from build123d import *

# Parameters (mm, degrees)
SKETCH_1_R          = 1.6
SKETCH_1_R_2        = 1.65
EXTRUDE_1_DEPTH     = 5
FILLET_1_R          = 2
SKETCH_2_R          = 3.5
CUT_EXTRUDE_1_DEPTH = 2.5
SKETCH_3_W          = 15.1
SKETCH_3_H          = 85
CUT_EXTRUDE_2_DEPTH = 1
SKETCH_4_R          = 1.25
CUT_EXTRUDE_3_DEPTH = 5
CHAMFER_1_SIZE      = 5
SKETCH_6_R          = 1.25
CUT_EXTRUDE_5_DEPTH = 5
SKETCH_7_R          = 1.25
CUT_EXTRUDE_6_DEPTH = 5
SKETCH_5_R          = 2.1
CUT_EXTRUDE_4_DEPTH = 6
CUT_EXTRUDE_7_DEPTH = 2.5
CUT_EXTRUDE_9_DEPTH = 6.0000001
SKETCH_9_W          = 33.95
SKETCH_9_H          = 29
CUT_EXTRUDE_8_DEPTH = 3.5
FILLET_29_R         = 2.1
FILLET_30_R         = 2


with BuildPart() as part:
    # ｽｹｯﾁ1 → ﾎﾞｽ - 押し出し1 (new body)
    with BuildSketch(Plane(origin=(0, 0, 0), x_dir=(1, 0, 0), z_dir=(0, 1, 0))):
        Polygon((-36.5, -42.5), (31.5, -42.5), (36.5, -32.5), (36.5, 32.5), (31.5, 42.5), (-36.5, 42.5), align=None)
        with Locations((-24, -18)):
            Circle(SKETCH_1_R, mode=Mode.SUBTRACT)
        with Locations((-24, 18)):
            Circle(SKETCH_1_R, mode=Mode.SUBTRACT)
        with Locations((24, 35)):
            Circle(SKETCH_1_R_2, mode=Mode.SUBTRACT)
        with Locations((24, -35)):
            Circle(SKETCH_1_R_2, mode=Mode.SUBTRACT)
        with Locations((24, -18)):
            Circle(SKETCH_1_R, mode=Mode.SUBTRACT)
        with Locations((24, 18)):
            Circle(SKETCH_1_R, mode=Mode.SUBTRACT)
    extrude(amount=EXTRUDE_1_DEPTH)

    # ﾌｨﾚｯﾄ1
    fillet_1_edges = [part.edges().sort_by_distance(p)[0] for p in [
        (31.5, 2.5, -42.5),
        (36.5, 2.5, -32.5),
        (36.5, 2.5, 32.5),
        (31.5, 2.5, 42.5),
    ]]
    fillet(fillet_1_edges, radius=FILLET_1_R)

    # ｽｹｯﾁ2 → ｶｯﾄ - 押し出し1 (cut)
    with BuildSketch(Plane(origin=(0, 5, 0), x_dir=(1, 0, 0), z_dir=(0, 1, 0))):
        with Locations((24, 18)):
            Circle(SKETCH_2_R)
        with Locations((24, -18)):
            Circle(SKETCH_2_R)
    extrude(amount=-CUT_EXTRUDE_1_DEPTH, mode=Mode.SUBTRACT)

    # ｽｹｯﾁ3 → ｶｯﾄ - 押し出し2 (cut)
    with BuildSketch(Plane(origin=(0, 5, 0), x_dir=(1, 0, 0), z_dir=(0, 1, 0))):
        with Locations((24, 0)):
            Rectangle(SKETCH_3_W, SKETCH_3_H)
    extrude(amount=-CUT_EXTRUDE_2_DEPTH, mode=Mode.SUBTRACT)

    # ｽｹｯﾁ4 → ｶｯﾄ - 押し出し3 (cut)
    with BuildSketch(Plane.ZY.offset(36.5)):
        with Locations((-35, 2.5)):
            Circle(SKETCH_4_R)
        with Locations((35, 2.5)):
            Circle(SKETCH_4_R)
    extrude(amount=-CUT_EXTRUDE_3_DEPTH, mode=Mode.SUBTRACT)

    # 面取り1
    chamfer_1_edges = [part.edges().sort_by_distance(p)[0] for p in [
        (-36.5, 2.5, 42.5),
        (-36.5, 2.5, -42.5),
    ]]
    chamfer(chamfer_1_edges, length=CHAMFER_1_SIZE)

    # ｽｹｯﾁ6 → ｶｯﾄ - 押し出し5 (cut)
    with BuildSketch(Plane.XY.offset(42.5)):
        with Locations((8.5, 2.5)):
            Circle(SKETCH_6_R)
    extrude(amount=-CUT_EXTRUDE_5_DEPTH, mode=Mode.SUBTRACT)

    # ｽｹｯﾁ7 → ｶｯﾄ - 押し出し6 (cut)
    with BuildSketch(Plane(origin=(0, 0, -42.5), x_dir=(-1, 0, 0), z_dir=(0, 0, -1))):
        with Locations((-8.5, 2.5)):
            Circle(SKETCH_7_R)
    extrude(amount=-CUT_EXTRUDE_6_DEPTH, mode=Mode.SUBTRACT)

    # ｽｹｯﾁ5 → ｶｯﾄ - 押し出し4 (cut, through all)
    with BuildSketch(Plane(origin=(0, 5, 0), x_dir=(1, 0, 0), z_dir=(0, 1, 0))):
        with Locations((-38.5, 35)):
            Circle(SKETCH_5_R)
        with Locations((-38.5, -35)):
            Circle(SKETCH_5_R)
        with Locations((8.5, -44.5)):
            Circle(SKETCH_5_R)
        with Locations((8.5, 44.5)):
            Circle(SKETCH_5_R)
    extrude(amount=-CUT_EXTRUDE_4_DEPTH, mode=Mode.SUBTRACT)

    # ｽｹｯﾁ8 → ｶｯﾄ - 押し出し7 (cut)
    with BuildSketch(Plane(origin=(0, 5, 0), x_dir=(1, 0, 0), z_dir=(0, 1, 0))):
        with BuildLine():
            Line((-20.5, 18), (-20.5, 21.5))
            Line((-20.5, 21.5), (-24, 21.5))
            ThreePointArc((-24, 21.5), (-26.474873734, 20.474873734), (-27.5, 18))
            Line((-27.5, 18), (-27.5, 14.5))
            Line((-27.5, 14.5), (-24, 14.5))
            ThreePointArc((-24, 14.5), (-21.525126266, 15.525126266), (-20.5, 18))
        make_face()
        with BuildLine():
            Line((-27.5, -18), (-27.5, -14.5))
            Line((-27.5, -14.5), (-24, -14.5))
            ThreePointArc((-24, -14.5), (-21.525126266, -15.525126266), (-20.5, -18))
            Line((-20.5, -18), (-20.5, -21.5))
            Line((-20.5, -21.5), (-24, -21.5))
            ThreePointArc((-24, -21.5), (-26.474873734, -20.474873734), (-27.5, -18))
        make_face()
    extrude(amount=-CUT_EXTRUDE_7_DEPTH, mode=Mode.SUBTRACT)

    # ｽｹｯﾁ10 → ｶｯﾄ - 押し出し9 (cut, through all)
    with BuildSketch(Plane(origin=(0, 5, 0), x_dir=(1, 0, 0), z_dir=(0, 1, 0))):
        with BuildLine():
            Line((-31.5, 32.5), (-31.5, 37.5))
            ThreePointArc((-31.5, 37.5), (-30, 39), (-28.5, 37.5))
            Line((-28.5, 37.5), (-28.5, 32.5))
            ThreePointArc((-28.5, 32.5), (-30, 31), (-31.5, 32.5))
        make_face()
        with BuildLine():
            Line((6, 37.5), (11, 37.5))
            ThreePointArc((11, 37.5), (12.5, 36), (11, 34.5))
            Line((11, 34.5), (6, 34.5))
            ThreePointArc((6, 34.5), (4.5, 36), (6, 37.5))
        make_face()
        with BuildLine():
            Line((6, -37.5), (11, -37.5))
            ThreePointArc((11, -37.5), (12.5, -36), (11, -34.5))
            Line((11, -34.5), (6, -34.5))
            ThreePointArc((6, -34.5), (4.5, -36), (6, -37.5))
        make_face()
        with BuildLine():
            Line((-31.5, -32.5), (-31.5, -37.5))
            ThreePointArc((-31.5, -37.5), (-30, -39), (-28.5, -37.5))
            Line((-28.5, -37.5), (-28.5, -32.5))
            ThreePointArc((-28.5, -32.5), (-30, -31), (-31.5, -32.5))
        make_face()
    extrude(amount=-CUT_EXTRUDE_9_DEPTH, mode=Mode.SUBTRACT)

    # ｽｹｯﾁ9 → ｶｯﾄ - 押し出し8 (cut)
    with BuildSketch(Plane(origin=(0, 5, 0), x_dir=(1, 0, 0), z_dir=(0, 1, 0))):
        with Locations((-3.525, 0)):
            Rectangle(SKETCH_9_W, SKETCH_9_H)
        with BuildLine():
            Line((-24, 21.5), (13.45, 21.5))
            Line((13.45, 21.5), (13.45, 34.5))
            Line((13.45, 34.5), (13.45, 37.5))
            Line((13.45, 37.5), (11, 37.5))
            Line((11, 37.5), (6, 37.5))
            Line((6, 37.5), (4.5, 37.5))
            Line((4.5, 37.5), (2.5, 39.5))
            Line((2.5, 39.5), (-31.5, 39.5))
            Line((-31.5, 39.5), (-31.5, 37.5))
            Line((-31.5, 37.5), (-31.5, 32.5))
            Line((-31.5, 32.5), (-31.5, 31))
            Line((-31.5, 31), (-33.5, 29))
            Line((-33.5, 29), (-33.5, -29))
            Line((-33.5, -29), (-31.5, -31))
            Line((-31.5, -31), (-31.5, -32.5))
            Line((-31.5, -32.5), (-31.5, -37.5))
            Line((-31.5, -37.5), (-31.5, -39.5))
            Line((-31.5, -39.5), (2.5, -39.5))
            Line((2.5, -39.5), (4.5, -37.5))
            Line((4.5, -37.5), (6, -37.5))
            Line((6, -37.5), (11, -37.5))
            Line((11, -37.5), (13.45, -37.5))
            Line((13.45, -37.5), (13.45, -34.5))
            Line((13.45, -34.5), (13.45, -21.5))
            Line((13.45, -21.5), (-24, -21.5))
            ThreePointArc((-24, -21.5), (-26.474873734, -20.474873734), (-27.5, -18))
            Line((-27.5, -18), (-27.5, 18))
            ThreePointArc((-27.5, 18), (-26.474873734, 20.474873734), (-24, 21.5))
        make_face()
    extrude(amount=-CUT_EXTRUDE_8_DEPTH, mode=Mode.SUBTRACT)

    # ﾌｨﾚｯﾄ29
    fillet_29_edges = [part.edges().sort_by_distance(p)[0] for p in [
        (13.45, 3.25, -21.5),
        (4.5, 3.25, -37.5),
        (13.45, 3.25, 37.5),
        (-31.5, 3.25, -31),
        (13.45, 3.25, 21.5),
        (4.5, 3.25, 37.5),
        (2.5, 3.25, 39.5),
        (-31.5, 3.25, 31),
        (-33.5, 3.25, 29),
        (-33.5, 3.25, -29),
        (2.5, 3.25, -39.5),
        (13.45, 3.25, -37.5),
        (-20.5, 3.25, 14.5),
        (-20.5, 3.25, -14.5),
        (13.45, 3.25, -14.5),
        (13.45, 3.25, 14.5),
    ]]
    fillet(fillet_29_edges, radius=FILLET_29_R)

    # ﾌｨﾚｯﾄ30
    fillet_30_edges = [part.edges().sort_by_distance(p)[0] for p in [
        (-31.5, 3.25, 39.5),
        (-31.5, 3.25, -39.5),
    ]]
    fillet(fillet_30_edges, radius=FILLET_30_R)


solid = part.part
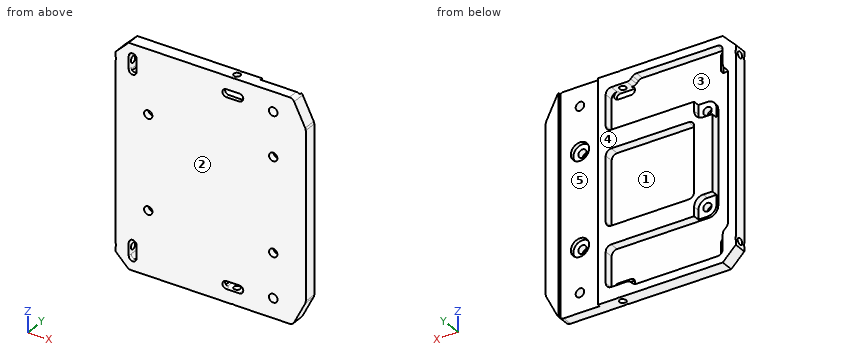
Geometry: final body of the model. Coordinates: model frame, mm. Face numbers are marked on the shaded views. A direction names the side the tool comes from. Round coordinates to 2 decimals unless told otherwise and drop trailing zeros. Loops run counter-clockwise (first coordinate to the right, second up) from the corner with the lowest first, then second, coordinate; pieces in that order, holes last.
Q1. Section A-A on z = 7.5. Return loops of the section in (x, y).
Q2. Pull-direction query (X, two-part tool) for the marked faces 3, 4 and 5; classes: released by +X, released by -X, zero draft, split by the parting line, or undercut.
Q3. Material intervals for L1, parallel to X at y = 1.85, z = 10; L2, parallel to Z at x = 24, y = 3.05; L3, parallel to X at y = 1.2, z = -18, sorted ascending.
Q4. Section B-B on x = -5. Return loops of the section in (y, z).
Q5. Pin query (flat end, axial travel): P1, Ø2.5, axis at x = -24, z = -18, coming from the +Y side; P2, Ø1.2, axis at y = 0.5, z = 35, coming from the -X side; P3, Ø2, axis at x = 22.5, z = -19, coming from the +Y side; P4, Ø8.5, axis at x = -0.5, z = -6.5, coming from the +Y side. Return the tip coordinate at first contact, or that it passes through.
Q6. Access query for the marked faces 1 and 2. Directions: +Z, -Z, +X, -X, +Y, -Y. A direction counts if a zero-diameter tool reaches every point of the face in a straight line with its end or side. Return the directions, or none.
Evaluation:
1. outline: (-36.5, 0) - (36.5, 0) - (36.5, 5) - (31.55, 5) - (31.55, 4) - (16.45, 4) - (16.45, 5) - (13.45, 5) - (13.45, 1.5) - (-20.5, 1.5) - (-20.5, 5) - (-27.5, 5) - (-27.5, 1.5) - (-33.5, 1.5) - (-33.5, 5) - (-36.5, 5) - close
2. face 3: undercut
2. face 4: zero draft
2. face 5: undercut
3. L1: x = -36.5 to -33.5, -27.5 to -20.5, 13.45 to 36.5
3. L2: z = -42.5 to -36.65, -33.35 to -21.5, -14.5 to 14.5, 21.5 to 33.35, 36.65 to 42.5
3. L3: x = -36.5 to -25.6, -22.4 to 22.4, 25.6 to 36.5
4. outline: (0, -42.5) - (5, -42.5) - (5, -39.5) - (1.5, -39.5) - (1.5, -21.5) - (5, -21.5) - (5, -14.5) - (1.5, -14.5) - (1.5, 14.5) - (5, 14.5) - (5, 21.5) - (1.5, 21.5) - (1.5, 39.5) - (5, 39.5) - (5, 42.5) - (0, 42.5) - close
5. P1: passes through
5. P2: stops at x = -36.49
5. P3: stops at y = 2.5
5. P4: stops at y = 1.5
6. face 1: +Y
6. face 2: +Z, -Z, +X, -X, -Y
